Input: part model. Units: mm. Frame: model coordinates. A direction names the side the tool comes from. Give positions to 0.01 mm unless a question says otherwise; leave off trailing zeros. Order: outer loops, then holes, each group sorted by start corner. A loop starts at its lowest first (then second) coordinate and runs counter-clockwise, first axis right, second up. Notation, with made-up numbers: (-8, 86.5) - (42, 86.5) arc R21 ccw to (42, 118.5) - close; hole circle Ø1 at (-25, 61.5). An arc over 180 degrees is marked (long way). Answer in a Markdown table with one row per item. Add a question column.
1. Contact query for flat-ended pins moving along their axis: pin 1 (2 mm diameter, centred on x = 13, y = -15, fed in from +Z); pin 2 (2 mm diameter, centred on y = -18, z = 20, fed in from -X); pin 3 (3.5 mm diameter, centred on x = 10.61, z = -10.61, fed in from +Y); pin 4 (1 mm diameter, centred on y = -12, z = -13.5, fed in from +X). Output: stop coordinate, or through.
2. Section query A-A on z = 0. Return loops of the section in (x, y), and give its area (3 significant figures).
3. Section query B-B on x = 0. Return loops of the section in (y, z).
4. Mould query, pull axis Z, two halves, no side actions, for faces 5 (the face through (-17.62, -12.325, -21.146)), 6 (the face through (2.507, -12.325, 27.341)), 7 (the face through (12.8, -12.3, -24.4)), 8 (the face through (6, 0, -6)). Classes: released by +Z, released by -Z, zero draft, split by the parting line, or undercut.
5. Access query for faces 1 (the face through (8, -12, -26)), 2 (the face through (-27.341, -12.325, 2.507)), 3 (the face through (27.412, -12.325, 2.493)), 4 (the face through (-4.851, -12.325, 24.525)). Directions: +Z, -Z, +X, -X, +Y, -Y. A direction counts if a zero-diameter tool reaches every point of the face in a straight line with its end or side. Return the directions, or none.
6. Section query D-D on x = -11. Return loops of the section in (y, z).
7. Section query C-C on y = -18.75. Count the separate pieces of the cut face and the enclosed holes in it, and give its area (3 significant figures).
8. Ray query, line 1 (Z direction, x = 0, y = -19.5); line 2 (Z direction, x = -26, y = -11.25); line 3 (X direction, y = -21, z = -27). Return the intervals inside material, ascending. Write a range as [from, to].
```python
from build123d import *

# Parameters (mm, degrees)
F0_R     = 3
F0_R_2   = 7.5
F1_DEPTH = 25


with BuildPart() as f1:
    # F0 (on Front) → F1 (new body)
    with BuildSketch(Plane.XZ):
        with BuildLine():
            Line((9.607203, 28.420092), (6.726314, 24.078137))
            ThreePointArc((6.726314, 24.078137), (4.877258, 24.519632), (3, 24.819347))
            Line((3, 24.819347), (2, 29.933259))
            Line((2, 29.933259), (-2, 29.933259))
            Line((-2, 29.933259), (-3, 24.819347))
            ThreePointArc((-3, 24.819347), (-4.877258, 24.519632), (-6.726314, 24.078137))
            Line((-6.726314, 24.078137), (-9.607203, 28.420092))
            Line((-9.607203, 28.420092), (-13.302721, 26.889359))
            Line((-13.302721, 26.889359), (-12.269592, 21.782037))
            ThreePointArc((-12.269592, 21.782037), (-13.889256, 20.78674), (-15.428608, 19.671249))
            Line((-15.428608, 19.671249), (-19.751797, 22.580224))
            Line((-19.751797, 22.580224), (-22.580224, 19.751797))
            Line((-22.580224, 19.751797), (-19.671249, 15.428608))
            ThreePointArc((-19.671249, 15.428608), (-20.78674, 13.889256), (-21.782037, 12.269592))
            Line((-21.782037, 12.269592), (-26.889359, 13.302721))
            Line((-26.889359, 13.302721), (-28.420092, 9.607203))
            Line((-28.420092, 9.607203), (-24.078137, 6.726314))
            ThreePointArc((-24.078137, 6.726314), (-24.519632, 4.877258), (-24.819347, 3))
            Line((-24.819347, 3), (-29.933259, 2))
            Line((-29.933259, 2), (-29.933259, -2))
            Line((-29.933259, -2), (-24.819347, -3))
            ThreePointArc((-24.819347, -3), (-24.519632, -4.877258), (-24.078137, -6.726314))
            Line((-24.078137, -6.726314), (-28.253115, -9.844271))
            Line((-28.253115, -9.844271), (-26.722382, -13.539789))
            Line((-26.722382, -13.539789), (-21.782037, -12.269592))
            ThreePointArc((-21.782037, -12.269592), (-20.78674, -13.889256), (-19.671249, -15.428608))
            Line((-19.671249, -15.428608), (-22.580224, -19.751797))
            Line((-22.580224, -19.751797), (-19.751797, -22.580224))
            Line((-19.751797, -22.580224), (-15.428608, -19.671249))
            ThreePointArc((-15.428608, -19.671249), (-13.889256, -20.78674), (-12.269592, -21.782037))
            Line((-12.269592, -21.782037), (-13.302721, -26.889359))
            Line((-13.302721, -26.889359), (-9.607203, -28.420092))
            Line((-9.607203, -28.420092), (-6.726314, -24.078137))
            ThreePointArc((-6.726314, -24.078137), (-4.877258, -24.519632), (-3, -24.819347))
            Line((-3, -24.819347), (-2, -29.933259))
            Line((-2, -29.933259), (2, -29.933259))
            Line((2, -29.933259), (3, -24.819347))
            ThreePointArc((3, -24.819347), (4.877258, -24.519632), (6.726314, -24.078137))
            Line((6.726314, -24.078137), (9.607203, -28.420092))
            Line((9.607203, -28.420092), (13.302721, -26.889359))
            Line((13.302721, -26.889359), (12.269592, -21.782037))
            ThreePointArc((12.269592, -21.782037), (13.889256, -20.78674), (15.428608, -19.671249))
            Line((15.428608, -19.671249), (19.751797, -22.580224))
            Line((19.751797, -22.580224), (22.580224, -19.751797))
            Line((22.580224, -19.751797), (19.671249, -15.428608))
            ThreePointArc((19.671249, -15.428608), (20.78674, -13.889256), (21.782037, -12.269592))
            Line((21.782037, -12.269592), (26.889359, -13.302721))
            Line((26.889359, -13.302721), (28.420092, -9.607203))
            Line((28.420092, -9.607203), (24.078137, -6.726314))
            ThreePointArc((24.078137, -6.726314), (24.519632, -4.877258), (24.819347, -3))
            Line((24.819347, -3), (29.933259, -2))
            Line((29.933259, -2), (29.933259, 2))
            Line((29.933259, 2), (24.819347, 3))
            ThreePointArc((24.819347, 3), (24.519632, 4.877258), (24.078137, 6.726314))
            Line((24.078137, 6.726314), (28.420092, 9.607203))
            Line((28.420092, 9.607203), (26.889359, 13.302721))
            Line((26.889359, 13.302721), (21.782037, 12.269592))
            ThreePointArc((21.782037, 12.269592), (20.78674, 13.889256), (19.671249, 15.428608))
            Line((19.671249, 15.428608), (22.580224, 19.751797))
            Line((22.580224, 19.751797), (19.751797, 22.580224))
            Line((19.751797, 22.580224), (15.428608, 19.671249))
            ThreePointArc((15.428608, 19.671249), (13.889256, 20.78674), (12.269592, 21.782037))
            Line((12.269592, 21.782037), (13.302721, 26.889359))
            Line((13.302721, 26.889359), (9.607203, 28.420092))
        make_face()
        with Locations((-15, 0)):
            Circle(F0_R, mode=Mode.SUBTRACT)
        with Locations((-5.740251, -13.858193)):
            Circle(F0_R, mode=Mode.SUBTRACT)
        Circle(F0_R_2, mode=Mode.SUBTRACT)
        with Locations((10.606602, -10.606602)):
            Circle(F0_R, mode=Mode.SUBTRACT)
        with Locations((0, 15)):
            Circle(F0_R, mode=Mode.SUBTRACT)
        with Locations((13.858193, 5.740251)):
            Circle(F0_R, mode=Mode.SUBTRACT)
    extrude(amount=F1_DEPTH)


solid = f1.part
```
Answer:
| question | item | result |
|---|---|---|
| 1 | pin 1 | stops at z = 27.43 |
| 1 | pin 2 | stops at x = -22.58 |
| 1 | pin 3 | passes through |
| 1 | pin 4 | stops at x = 27.01 |
| 2 | outline | (-29.93, -25) - (-18, -25) - (-18, 0) - (-29.93, 0) - close; (-12, -25) - (-7.5, -25) - (-7.5, 0) - (-12, 0) - close; (7.5, -25) - (29.93, -25) - (29.93, 0) - (7.5, 0) - close |
| 2 | area | 972 mm² |
| 3 | outline | (-25, -29.93) - (0, -29.93) - (0, -7.5) - (-25, -7.5) - close; (-25, 7.5) - (0, 7.5) - (0, 12) - (-25, 12) - close; (-25, 18) - (0, 18) - (0, 29.93) - (-25, 29.93) - close |
| 4 | face 5 | released by -Z |
| 4 | face 6 | released by +Z |
| 4 | face 7 | undercut |
| 4 | face 8 | zero draft |
| 5 | face 1 | -Z, +Y, -Y |
| 5 | face 2 | -X, +Y, -Y |
| 5 | face 3 | +X, +Y, -Y |
| 5 | face 4 | +Z, +Y, -Y |
| 6 | outline | (-25, -27.84) - (0, -27.84) - (0, 27.84) - (-25, 27.84) - close |
| 7 | separate pieces | 1 |
| 7 | enclosed holes | 6 |
| 7 | area | 2,040 mm² |
| 8 | line 1 | z = [-29.93, -7.5], [7.5, 12], [18, 29.93] |
| 8 | line 2 | z = [-13.35, -8.16], [-2.77, 2.77], [8, 13.12] |
| 8 | line 3 | x = [-13.04, -8.66], [-2.57, 2.57], [8.66, 13.04] |
